```python
from build123d import *

# Parameters (mm, degrees)
AUFSATZ_LINEAR_AUSTRAGEN1_DEPTH = 20
SKIZZE2_W                       = 11
SKIZZE2_H                       = 5
SCHNITT_LINEAR_AUSTRAGEN1_DEPTH = 0.5
AUFSATZ_LINEAR_AUSTRAGEN2_DEPTH = 8
SKIZZE4_W                       = 1.5
SKIZZE4_H                       = 2
SCHNITT_LINEAR_AUSTRAGEN2_DEPTH = 8
AUFSATZ_LINEAR_AUSTRAGEN3_DEPTH = 2.5
SKIZZE8_W                       = 3
SKIZZE8_H                       = 12.320508076
SCHNITT_LINEAR_AUSTRAGEN5_DEPTH = 12
SKIZZE9_W                       = 9.95
SKIZZE9_H                       = 5.773502692
SKIZZE9_W_2                     = 10
AUFSATZ_LINEAR_AUSTRAGEN5_DEPTH = 0.5
AUFSATZ_LINEAR_AUSTRAGEN6_DEPTH = 2.5


with BuildPart() as part:
    # Skizze1 → Aufsatz-Linear austragen1 (new body)
    with BuildSketch(Plane(origin=(0, 0, 0), x_dir=(1, 0, 0), z_dir=(0, 1, 0))):
        Polygon((1.5, 2.5), (1.5, 5), (12.5, 5), (12.5, 2.5), (14.5, 2.5), (14.5, -0.5), (12.5, -0.5), (12.5, -3), (1.5, -3), (1.5, -0.5), (-0.5, -0.5), (-0.5, 2.5), align=None)
        Polygon((2, 2), (2, 4.5), (12, 4.5), (12, 2), (14, 2), (14, 0), (12, 0), (12, -2.5), (2, -2.5), (2, 0), (0, 0), (0, 2), align=None, mode=Mode.SUBTRACT)
    extrude(amount=AUFSATZ_LINEAR_AUSTRAGEN1_DEPTH)

    # Skizze2 → Schnitt-Linear austragen1 (cut)
    with BuildSketch(Plane(origin=(0, 0, -5), x_dir=(-1, 0, 0), z_dir=(0, 0, -1))):
        with Locations((-7, 17.5)):
            Rectangle(SKIZZE2_W, SKIZZE2_H)
    extrude(amount=-SCHNITT_LINEAR_AUSTRAGEN1_DEPTH, mode=Mode.SUBTRACT)

    # Skizze3 → Aufsatz-Linear austragen2 (add)
    with BuildSketch(Plane(origin=(0, 0, -5), x_dir=(-1, 0, 0), z_dir=(0, 0, -1))):
        Polygon((-1.5, 0), (0.5, 0), (10.5, -17.320508076), (10.933012702, -17.070508076), (0.788675135, 0.5), (-1.5, 0.5), align=None)
    extrude(amount=-AUFSATZ_LINEAR_AUSTRAGEN2_DEPTH)

    # Skizze4 → Schnitt-Linear austragen2 (cut)
    with BuildSketch(Plane(origin=(0, 0.5, 0), x_dir=(1, 0, 0), z_dir=(0, 1, 0))):
        with Locations((0.75, 1)):
            Rectangle(SKIZZE4_W, SKIZZE4_H)
    extrude(amount=-SCHNITT_LINEAR_AUSTRAGEN2_DEPTH, mode=Mode.SUBTRACT)

    # Skizze6 → Aufsatz-Linear austragen3 (add)
    with BuildSketch(Plane(origin=(0, 0, -5), x_dir=(-1, 0, 0), z_dir=(0, 0, -1))):
        Polygon((-1.5, 15), (10.933012702, -17.070508076), (0.788675135, 0.5), (-1.5, 0.5), align=None)
    extrude(amount=-AUFSATZ_LINEAR_AUSTRAGEN3_DEPTH)

    # Skizze8 → Schnitt-Linear austragen5 (cut)
    with BuildSketch(Plane(origin=(0, 0, 0), x_dir=(0, 0, -1), z_dir=(1, 0, 0))):
        with Locations((1, -6.160254038)):
            Rectangle(SKIZZE8_W, SKIZZE8_H)
    extrude(amount=-SCHNITT_LINEAR_AUSTRAGEN5_DEPTH, mode=Mode.SUBTRACT)

    # Skizze9 → Aufsatz-Linear austragen5 (add)
    with BuildSketch(Plane(origin=(-0.375, 0.216506351, 0), x_dir=(0, 0, -1), z_dir=(0.866025404, -0.5, 0))):
        with Locations((-7.975, -17.363248654)):
            Rectangle(SKIZZE9_W, SKIZZE9_H)
        with Locations((10, -17.363248654)):
            Rectangle(SKIZZE9_W_2, SKIZZE9_H)
    extrude(amount=-AUFSATZ_LINEAR_AUSTRAGEN5_DEPTH)

    # Skizze11 → Aufsatz-Linear austragen6 (add)
    with BuildSketch(Plane.XY.offset(0.5)):
        Polygon((1.5, 0.5), (-0.788675135, 0.5), (-10.933012702, -17.070508076), (1.5, 15), align=None)
    extrude(amount=AUFSATZ_LINEAR_AUSTRAGEN6_DEPTH)


solid = part.part
```
Can you work these out from the model? Positions are in its coordinate system, mm. A direction names the side the tool comes from. Round coordinates to 2 decimals unless told otherwise and drop trailing zeros. Order: outer loops, then holes, each group sorted by start corner. A loop starts at its lowest first (then second) coordinate and runs counter-clockwise, first axis right, second up. Notation, with made-up numbers: (-25, -18) -> (-10, -18) arc R16 ccw to (-10, -13) -> close; hole circle Ø11 at (84, 83). An arc over 180 degrees is marked (long way). Return JSON: item names as keys, results as strings. Group by question number.
1. I need wall thicknesses on line 1 (Z direction, x = 8, y = 1); line 2 (Z direction, x = -3, y = 3); line 3 (X direction, y = -10, z = -4.75). Which ranges of each line are inside material? Lowest first, please. Write a range as [from, to].
2. Which directions (+Z, -Z, +X, -X, +Y, -Y) give clear straight access to the entire face, cutting with the end or side of a thin tool? Please do faces 1 (the face through (-0.5, 10, -1)), 2 (the face through (-4.63, -0.81, -3.77)), 3 (the face through (14, 10, 0.5)), 4 (the face through (13, 10, -2)), 5 (the face through (12.5, 10, -4)).
3. If we section it at B-B, the plane x = 3: Write out the boundary of the cut face in (y, z).
4. If we section it at A-A, the plane y = -0.5: Write out the boundary of the cut face in (x, z), then the cut area to 3 significant figures.
5. Will these pins go through, and if not, where does the flat tip stop? pin 1 (3 mm diameter, centred on x = -7.5, y = -8, fed in from +Z); pin 2 (0.6 mm diameter, centred on x = -8, z = -0.5, fed in from +Y); pin 3 (6 mm diameter, centred on x = 10.5, z = -0.5, fed in from -Y); pin 4 (12 mm diameter, centred on x = -6.5, y = -13.5, fed in from +Z).
6. If we section it at C-C, the plane y = 3.5: Write out the boundary of the cut face in (x, z).
7. If we section it at D-D, the plane y = -14: Write out the boundary of the cut face in (x, z).
Output values:
{
 "1": {"line 1": "[-5, -4.5], [2.5, 3]", "line 2": "[-5, -2.5], [0.5, 3]", "line 3": "[-8.19, -6.27]"},
 "2": {"face 1": "-X, +Y", "face 2": "-Z, -X, +Y", "face 3": "+Z, +X, +Y, -Y", "face 4": "+Y, -Y", "face 5": "-Z, +X, +Y, -Y"},
 "3": {"outline": "(0, -5) -> (15, -5) -> (15, -4.5) -> (0, -4.5) -> close; (0, 2.5) -> (20, 2.5) -> (20, 3) -> (0, 3) -> close"},
 "4": {"outline": "(-4.51, -5) -> (-0.79, -5) -> (-0.79, -2.5) -> (-4.51, -2.5) -> close; (-4.51, 0.5) -> (-0.79, 0.5) -> (-0.79, 3) -> (-4.51, 3) -> close", "area": "18.6 mm²"},
 "5": {"pin 1": "z = 3", "pin 2": "y = -12.32", "pin 3": "y = 0", "pin 4": "z = 12.95"},
 "6": {"outline": "(-2.96, -5) -> (12.5, -5) -> (12.5, -2.5) -> (14.5, -2.5) -> (14.5, 0.5) -> (12.5, 0.5) -> (12.5, 3) -> (-2.96, 3) -> (-2.96, 0.5) -> (-0.5, 0.5) -> (-0.5, -2.5) -> (-2.96, -2.5) -> close; hole (0, -2) -> (2, -2) -> (2, -4.5) -> (12, -4.5) -> (12, -2) -> (14, -2) -> (14, 0) -> (12, 0) -> (12, 2.5) -> (2, 2.5) -> (2, 0) -> (0, 0) -> close"},
 "7": {"outline": "(-9.74, -5) -> (-9.16, -5) -> (-9.16, -15) -> (-8.58, -15) -> (-8.58, 12.95) -> (-9.16, 12.95) -> (-9.16, 3) -> (-9.74, 3) -> (-9.74, 0.5) -> (-9.16, 0.5) -> (-9.16, -2.5) -> (-9.74, -2.5) -> close"}
}
